from build123d import *

# Parameters (mm, degrees)
F2_R     = 4
F3_DEPTH = 20.418424405
F4_R     = 1.75
F5_DEPTH = 25
F2_R_2   = 5
F6_DEPTH = 25
F7_DEPTH = 10


with BuildPart() as f1:
    # F0 (on Front) → F1 (revolve)
    with BuildSketch(Plane.XZ):
        with BuildLine():
            Line((30.9380175069, 2.5), (30.9380175069, 0))
            Line((30.9380175069, 0), (32.0326841507, 0))
            Line((32.0326841507, 0), (50.9380175069, 0))
            Line((50.9380175069, 0), (50.9380175069, 16.5))
            Line((50.9380175069, 16.5), (30.9380175069, 16.5))
            Line((30.9380175069, 16.5), (9, 16.5))
            Line((9, 16.5), (0, 16.5))
            Line((0, 16.5), (0, 1.875))
            Line((0, 1.875), (9, 1.875))
            Line((9, 1.875), (9, 2.5))
            ThreePointArc((9, 2.5), (10.4644660941, 6.0355339059), (14, 7.5))
            Line((14, 7.5), (25.9380175069, 7.5))
            ThreePointArc((25.9380175069, 7.5), (29.4735514129, 6.0355339059), (30.9380175069, 2.5))
        make_face()
    revolve(axis=Axis((16.0163420754, 0, 0), (1, 0, 0)))

    # F2 (on face) → F3 (cut, through all)
    with BuildSketch(Plane.YZ.offset(50.9380175069)):
        with Locations((0, 0.5)):
            Circle(F2_R)
    extrude(amount=-F3_DEPTH, mode=Mode.SUBTRACT)

    # F4 (on Front) → F5 (cut)
    with BuildSketch(Plane.XZ):
        with Locations((43.1880175069, 0.5)):
            Circle(F4_R)
    extrude(amount=-F5_DEPTH, mode=Mode.SUBTRACT)

    # F2 (on face) → F6 (cut)
    with BuildSketch(Plane.YZ.offset(50.9380175069)):
        with Locations((0, 0.5)):
            Circle(F2_R_2)
        with Locations((0, 0.5)):
            Circle(F2_R, mode=Mode.SUBTRACT)
    extrude(amount=-F6_DEPTH, mode=Mode.SUBTRACT)

    # F2 (on face) → F7 (join)
    with BuildSketch(Plane.YZ.offset(50.9380175069)):
        with Locations((0, 0.5)):
            Circle(F2_R_2)
        with Locations((0, 0.5)):
            Circle(F2_R, mode=Mode.SUBTRACT)
    extrude(amount=-F7_DEPTH)


solid = f1.part
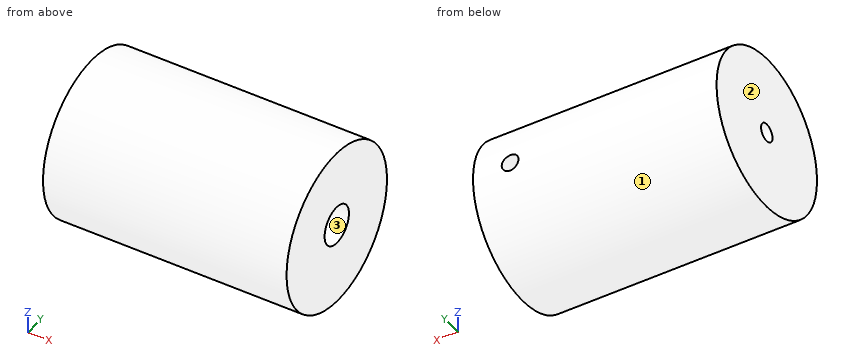
Check sheet for the modelled part. Datum: model origin and axes. Units: mm. Face numbers are marked on the shaded views. Round coordinates to 2 decimals unless told otherwise and drop trailing zeros. Loops run counter-clockwise (first coordinate to the right, second up) from the corner with the lowest first, then second, coordinate; pieces in that order, holes last. Notation, with made-up numbers: (24, 39) -> (79, 39) arc R20 ccw to (79, 52) -> close; hole circle Ø7 at (1.25, -30.5). An arc over 180 degrees is marked (long way). Put each result on its own line as item: value. Start each with the question number.
1. Gauge pin test, flat ends, axial feed: pin 1 (17 mm diameter, centred on y = 0, z = 0, fed in from -X); pin 2 (6.5 mm diameter, centred on y = 0, z = 0.5, fed in from +X); pin 3 (6 mm diameter, centred on x = 39, z = -5.5, fed in from +Y); pin 4 (2.5 mm diameter, centred on y = 1, z = -0.5, fed in from +X). Record the tip position at first contact, or that the pin passes through.
2. Section check B-B (y = 11.5). Enter the section's corners in (x, z), plus the area to 3 significant figures.
3. Section check D-D (y = -11.5). Enter the section's corners in (x, z), plus the area to 3 significant figures.
4. Draft check along Z on the marked faces 1, 2 and 3. Enter one of: +Z half, -Z half, draft (parallel to the pull), parting line (faces both ways), or undercut.
5. Section check A-A (x = 4). Enter the section's corners in (y, z) (3 decimals).
6. Section check C-C (z = -12.5). Enter the section's corners in (x, y).
7. Scan lines: probe 1 along Z at (x, y) = (44.25, 0); probe 2 along Y at (x, z) = (5, 0) (3 decimals); probe 3 along Z at (x, y) = (21, 0). Record each from-to range of solid material in increasing order.
Findings:
1. pin 1: stops at x = 0
1. pin 2: stops at x = 9.16
1. pin 3: stops at y = 16.31
1. pin 4: stops at x = 9
2. outline: (0, -11.83) -> (50.94, -11.83) -> (50.94, 11.83) -> (0, 11.83) -> close; hole circle Ø3.5 at (43.19, 0.5)
2. area: 1,200 mm^2
3. outline: (0, -11.83) -> (50.94, -11.83) -> (50.94, 11.83) -> (0, 11.83) -> close
3. area: 1,210 mm^2
4. face 1: parting line
4. face 2: draft
4. face 3: undercut
5. outline: circle Ø33 at (0, 0); hole circle Ø3.75 at (0, 0)
6. outline: (0, -10.77) -> (50.94, -10.77) -> (50.94, 10.77) -> (0, 10.77) -> close
7. probe 1: z = -16.5 to -3.5, 4.5 to 16.5
7. probe 2: y = -16.5 to -1.875, 1.875 to 16.5
7. probe 3: z = -16.5 to -7.5, 7.5 to 16.5
